CAD build for the part. Positions are in the model's coordinates, mm. A direction names the side the tool comes from. Give positions to 0.01 mm unless a question says otherwise; leave off trailing zeros. Write each loop counter-clockwise with the first axis right and the second up, starting at its lowest first coordinate (ties: lowest second). Pieces come first, ordered by that corner, then holes. Notation, with made-up numbers: (68.25, 27.25) -> (90.25, 27.25) arc R21 ccw to (90.25, 52.25) -> close; hole circle Ø7 at (-23.75, 56.25). An arc over 180 degrees is marked (long way). Answer as a JSON object with one key per item and string values.
```python
from build123d import *

# Parameters (mm, degrees)
BOSS_EXTRUDE1_DEPTH  = 5
EDGE_FLANGE1_START   = -417.4
EDGE_FLANGE1_DEPTH   = 834.8
EDGE_FLANGE1_START_2 = -419.24
EDGE_FLANGE1_2_DEPTH = 838.48
EDGE_FLANGE1_3_DEPTH = 834.8
EDGE_FLANGE1_4_DEPTH = 838.48
BOSS_EXTRUDE2_START  = -20
BOSS_EXTRUDE2_DEPTH  = 20
BOSS_EXTRUDE6_START  = -20
BOSS_EXTRUDE6_DEPTH  = 20
MIRROR2_START        = -20
MIRROR2_COPY_1_DEPTH = 20
MIRROR2_COPY_2_DEPTH = 20
BOSS_EXTRUDE7_DEPTH  = 20
CUT_EXTRUDE1_REACH   = 921.649
SKETCH21_R           = 9.25
BOSS_EXTRUDE8_REACH  = 918.804
SKETCH22_R           = 150
SKETCH23_R           = 145
CUT_EXTRUDE2_DEPTH   = 920.648675088
FILLET1_R            = 10


# Read off the part's stored shape, not the designer's step: Edge-Flange1
with BuildPart() as part:
    # Sketch1 → Boss-Extrude1 (new body)
    with BuildSketch(Plane(origin=(0, 0, 0), x_dir=(1, 0, 0), z_dir=(0, 1, 0))):
        Polygon((-419.24, -417.4), (-419.24, -582.5), (419.24, -582.5), (419.24, -417.4), (482.5, -417.4), (482.5, 417.4), (419.24, 417.4), (419.24, 582.5), (-419.24, 582.5), (-419.24, 417.4), (-482.5, 417.4), (-482.5, -417.4), align=None)
    extrude(amount=BOSS_EXTRUDE1_DEPTH)

    # Edge-Flange1 outline → Edge-Flange1 (add)
    with BuildSketch(Plane.XY.offset(EDGE_FLANGE1_START)):
        with BuildLine():
            Line((-479.84720202, 35.321619656), (-481.510736273, 16.307336141))
            ThreePointArc((-481.510736273, 16.307336141), (-480.800529715, 10.26398325), (-477.748155652, 4.999999958))
            Line((-477.748155652, 4.999999958), (-466.567815802, 5))
            ThreePointArc((-466.567815802, 5), (-473.94058917, 8.244097924), (-476.529762783, 15.871557427))
            Line((-476.529762783, 15.871557427), (-474.86622853, 34.885840943))
            Line((-474.86622853, 34.885840943), (-479.84720202, 35.321619656))
        make_face()
        with BuildLine():
            ThreePointArc((476.529762783, 15.871557427), (473.94058917, 8.244097924), (466.567815802, 5))
            Line((466.567815802, 5), (477.748155652, 4.999999958))
            ThreePointArc((477.748155652, 4.999999958), (480.800529715, 10.26398325), (481.510736273, 16.307336141))
            Line((481.510736273, 16.307336141), (479.84720202, 35.321619656))
            Line((479.84720202, 35.321619656), (474.86622853, 34.885840943))
            Line((474.86622853, 34.885840943), (476.529762783, 15.871557427))
        make_face()
    extrude(amount=EDGE_FLANGE1_DEPTH)

    # Edge-Flange1 2 outline → Edge-Flange1 2 (add)
    with BuildSketch(Plane.YZ.offset(EDGE_FLANGE1_START_2)):
        with BuildLine():
            Line((35.321619656, 579.84720202), (16.307336141, 581.510736273))
            ThreePointArc((16.307336141, 581.510736273), (10.263983245, 580.800529713), (4.99999995, 577.748155645))
            Line((4.99999995, 577.748155645), (5, 566.567815802))
            ThreePointArc((5, 566.567815802), (8.244097924, 573.94058917), (15.871557427, 576.529762783))
            Line((15.871557427, 576.529762783), (34.885840943, 574.86622853))
            Line((34.885840943, 574.86622853), (35.321619656, 579.84720202))
        make_face()
        with BuildLine():
            ThreePointArc((15.871557427, -576.529762783), (8.244097924, -573.94058917), (5, -566.567815802))
            Line((5, -566.567815802), (4.99999995, -577.748155645))
            ThreePointArc((4.99999995, -577.748155645), (10.263983245, -580.800529713), (16.307336141, -581.510736273))
            Line((16.307336141, -581.510736273), (35.321619656, -579.84720202))
            Line((35.321619656, -579.84720202), (34.885840943, -574.86622853))
            Line((34.885840943, -574.86622853), (15.871557427, -576.529762783))
        make_face()
    extrude(amount=EDGE_FLANGE1_2_DEPTH)

    # Edge-Flange1 3 outline → Edge-Flange1 3 (cut)
    with BuildSketch(Plane.XY.offset(EDGE_FLANGE1_START)):
        with BuildLine():
            ThreePointArc((-466.567815802, 0), (-472.691540133, 1.306936051), (-477.748155652, 4.999999958))
            Line((-477.748155652, 4.999999958), (-483, 4.999999958))
            Line((-483, 4.999999958), (-483, -2.2e-08))
            Line((-483, -2.2e-08), (-466.567815802, 0))
        make_face()
        with BuildLine():
            ThreePointArc((477.748155652, 4.999999958), (472.691540133, 1.306936051), (466.567815802, 0))
            Line((466.567815802, 0), (483, -2.2e-08))
            Line((483, -2.2e-08), (483, 4.999999958))
            Line((483, 4.999999958), (477.748155652, 4.999999958))
        make_face()
    extrude(amount=EDGE_FLANGE1_3_DEPTH, mode=Mode.SUBTRACT)

    # Edge-Flange1 4 outline → Edge-Flange1 4 (cut)
    with BuildSketch(Plane.YZ.offset(EDGE_FLANGE1_START_2)):
        with BuildLine():
            ThreePointArc((0, 566.567815802), (1.306936049, 572.691540128), (4.99999995, 577.748155645))
            Line((4.99999995, 577.748155645), (4.99999995, 583))
            Line((4.99999995, 583), (-2.7e-08, 583))
            Line((-2.7e-08, 583), (0, 566.567815802))
        make_face()
        with BuildLine():
            ThreePointArc((4.99999995, -577.748155645), (1.306936049, -572.691540128), (0, -566.567815802))
            Line((0, -566.567815802), (-2.7e-08, -583))
            Line((-2.7e-08, -583), (4.99999995, -583))
            Line((4.99999995, -583), (4.99999995, -577.748155645))
        make_face()
    extrude(amount=EDGE_FLANGE1_4_DEPTH, mode=Mode.SUBTRACT)

    # Sketch18 → Boss-Extrude2 (add)
    with BuildSketch(Plane(origin=(419.24, 0, 0), x_dir=(0, 0, -1), z_dir=(1, 0, 0)).offset(BOSS_EXTRUDE2_START)):
        with BuildLine():
            Line((-417.4, 5), (-566.567815802, 5))
            ThreePointArc((-566.567815802, 5), (-573.94058917, 8.244097924), (-576.529762783, 15.871557427))
            Line((-576.529762783, 15.871557427), (-533.736569049, 505))
            Line((-533.736569049, 505), (-417.4, 505))
            Line((-417.4, 505), (-417.4, 5))
        make_face()
    boss_extrude2 = extrude(amount=BOSS_EXTRUDE2_DEPTH)

    # Sketch19 → Boss-Extrude6 (add)
    with BuildSketch(Plane.XY.offset(417.4).offset(BOSS_EXTRUDE6_START)):
        with BuildLine():
            Line((466.567815802, 5), (419.24, 5))
            Line((419.24, 5), (399.24, 5))
            Line((399.24, 5), (399.24, 505))
            Line((399.24, 505), (419.24, 505))
            Line((419.24, 505), (433.736569049, 505))
            Line((433.736569049, 505), (476.529762783, 15.871557427))
            ThreePointArc((476.529762783, 15.871557427), (473.94058917, 8.244097924), (466.567815802, 5))
        make_face()
    boss_extrude6 = extrude(amount=BOSS_EXTRUDE6_DEPTH)

    # Mirror1: Boss-Extrude2, Boss-Extrude6 across plane
    add(boss_extrude2.mirror(Plane.XY))
    add(boss_extrude6.mirror(Plane.XY))

    # Mirror2: Boss-Extrude2, Boss-Extrude6 across plane
    add(boss_extrude2.mirror(Plane(origin=(0, 0, 0), x_dir=(0, 0, 1), z_dir=(1, 0, 0))))
    add(boss_extrude6.mirror(Plane(origin=(0, 0, 0), x_dir=(0, 0, 1), z_dir=(1, 0, 0))))

    # Mirror2 copy 1 sketch → Mirror2 copy 1 (add)
    with BuildSketch(Plane.ZY.offset(419.24).offset(MIRROR2_START)):
        with BuildLine():
            Line((-417.4, 5), (-566.567815802, 5))
            ThreePointArc((-566.567815802, 5), (-573.94058917, 8.244097924), (-576.529762783, 15.871557427))
            Line((-576.529762783, 15.871557427), (-533.736569049, 505))
            Line((-533.736569049, 505), (-417.4, 505))
            Line((-417.4, 505), (-417.4, 5))
        make_face()
    extrude(amount=MIRROR2_COPY_1_DEPTH)

    # Mirror2 copy 2 sketch → Mirror2 copy 2 (add)
    with BuildSketch(Plane(origin=(0, 0, -417.4), x_dir=(-1, 0, 0), z_dir=(0, 0, -1)).offset(MIRROR2_START)):
        with BuildLine():
            Line((466.567815802, 5), (419.24, 5))
            Line((419.24, 5), (399.24, 5))
            Line((399.24, 5), (399.24, 505))
            Line((399.24, 505), (419.24, 505))
            Line((419.24, 505), (433.736569049, 505))
            Line((433.736569049, 505), (476.529762783, 15.871557427))
            ThreePointArc((476.529762783, 15.871557427), (473.94058917, 8.244097924), (466.567815802, 5))
        make_face()
    extrude(amount=MIRROR2_COPY_2_DEPTH)

    # Sketch20 → Boss-Extrude7 (add)
    with BuildSketch(Plane(origin=(0, 505, 0), x_dir=(1, 0, 0), z_dir=(0, 1, 0))):
        Polygon((-419.24, -417.4), (-419.24, -533.736569049), (419.24, -533.736569049), (419.24, -417.4), (433.736569049, -417.4), (433.736569049, 417.4), (419.24, 417.4), (419.24, 533.736569049), (-419.24, 533.736569049), (-419.24, 417.4), (-433.736569049, 417.4), (-433.736569049, -417.4), align=None)
    extrude(amount=BOSS_EXTRUDE7_DEPTH)

    # Sketch21 → Cut-Extrude1 (cut, up to next)
    with BuildSketch(Plane(origin=(0, 525, 0), x_dir=(1, 0, 0), z_dir=(0, 1, 0)), mode=Mode.PRIVATE) as cut_extrude1_sk1:
        with Locations(Location((0, -249.998440062, 0), (0, 0, 270))):
            Circle(SKETCH21_R)
    cut_extrude1_tool1 = extrude(cut_extrude1_sk1.sketch, amount=-CUT_EXTRUDE1_REACH, mode=Mode.PRIVATE) & part.part
    # Sketch21 → Cut-Extrude1 (cut, up to next)
    with BuildSketch(Plane(origin=(0, 525, 0), x_dir=(1, 0, 0), z_dir=(0, 1, 0)), mode=Mode.PRIVATE) as cut_extrude1_sk2:
        with Locations(Location((-216.505, 124.999220031, 0), (0, 0, 270))):
            Circle(SKETCH21_R)
    cut_extrude1_tool2 = extrude(cut_extrude1_sk2.sketch, amount=-CUT_EXTRUDE1_REACH, mode=Mode.PRIVATE) & part.part
    # Sketch21 → Cut-Extrude1 (cut, up to next)
    with BuildSketch(Plane(origin=(0, 525, 0), x_dir=(1, 0, 0), z_dir=(0, 1, 0)), mode=Mode.PRIVATE) as cut_extrude1_sk3:
        with Locations(Location((216.505, 124.999220031, 0), (0, 0, 270))):
            Circle(SKETCH21_R)
    cut_extrude1_tool3 = extrude(cut_extrude1_sk3.sketch, amount=-CUT_EXTRUDE1_REACH, mode=Mode.PRIVATE) & part.part
    add(cut_extrude1_tool1.solids().sort_by_distance((0, 525, 249.99844))[0], mode=Mode.SUBTRACT)
    add(cut_extrude1_tool2.solids().sort_by_distance((-216.505, 525, -124.99922))[0], mode=Mode.SUBTRACT)
    add(cut_extrude1_tool3.solids().sort_by_distance((216.505, 525, -124.99922))[0], mode=Mode.SUBTRACT)

    # Sketch22 → Boss-Extrude8 (add, up to next)
    with BuildSketch(Plane(origin=(0, 5, 0), x_dir=(1, 0, 0), z_dir=(0, 1, 0)), mode=Mode.PRIVATE) as boss_extrude8_sk1:
        with Locations(Location((0, 0, 0), (0, 0, 270))):
            Circle(SKETCH22_R)
    boss_extrude8_tool1 = extrude(boss_extrude8_sk1.sketch, amount=BOSS_EXTRUDE8_REACH, mode=Mode.PRIVATE) - part.part
    add(boss_extrude8_tool1.solids().sort_by_distance((0, 5, 0))[0])

    # Sketch23 → Cut-Extrude2 (cut, through all)
    with BuildSketch(Plane(origin=(0, 525, 0), x_dir=(1, 0, 0), z_dir=(0, 1, 0))):
        with Locations(Location((0, 0, 0), (0, 0, 270))):
            Circle(SKETCH23_R)
    extrude(amount=-CUT_EXTRUDE2_DEPTH, mode=Mode.SUBTRACT)

    # Fillet1
    fillet1_edges = [part.edges().sort_by_distance(p)[0] for p in [
        (0, 505, -150),
        (0, 5, -150),
    ]]
    fillet(fillet1_edges, radius=FILLET1_R)


solid = part.part
```
1) Slice it at C-C (y = 367.5). List the corners of the cut face in (x, z), then the cut area to 3 significant figures.
Model answer:
{"outline": "(-445.77, -417.4) -> (-419.24, -417.4) -> (-419.24, -545.77) -> (-399.24, -545.77) -> (-399.24, -397.4) -> (-445.77, -397.4) -> close; (-445.77, 397.4) -> (-399.24, 397.4) -> (-399.24, 545.77) -> (-419.24, 545.77) -> (-419.24, 417.4) -> (-445.77, 417.4) -> close; circle Ø300 at (0, 0); (399.24, -545.77) -> (419.24, -545.77) -> (419.24, -417.4) -> (445.77, -417.4) -> (445.77, -397.4) -> (399.24, -397.4) -> close; (399.24, 397.4) -> (445.77, 397.4) -> (445.77, 417.4) -> (419.24, 417.4) -> (419.24, 545.77) -> (399.24, 545.77) -> close; hole circle Ø290 at (0, 0)", "area": "18,600 mm2"}
2) Slice it at A-A (z = -206). List the corners of the cut face in (x, y), then the cut area to 3 significant figures.
Model answer:
{"outline": "(-481.51, 16.31) arc R15 ccw to (-466.57, 0) -> (466.57, 0) arc R15 ccw to (481.51, 16.31) -> (479.85, 35.32) -> (474.87, 34.89) -> (476.53, 15.87) arc R10 cw to (466.57, 5) -> (-466.57, 5) arc R10 cw to (-476.53, 15.87) -> (-474.87, 34.89) -> (-479.85, 35.32) -> close; (-433.74, 505) -> (433.74, 505) -> (433.74, 525) -> (-433.74, 525) -> close", "area": "22,400 mm2"}
3) Mould opens along Z. For faces 3 (the flat face through (419.24, 259, -480)), 4 (the cylindrical face through (43.554, 266.175, 138.304)), 5 (the flat face through (-409.1, 266.65, -554.59)), 6 (the flat face through (-110, 5, -134)) say: released by +Z, released by -Z, zero draft, split by the parting line, or undercut.
Model answer:
{"face 3": "zero draft", "face 4": "undercut", "face 5": "released by -Z", "face 6": "undercut"}
4) Slice it at B-B (x = 270.5). List the corners of the cut face in (y, z).
Model answer:
{"outline": "(0, -566.57) arc R15 ccw to (16.31, -581.51) -> (35.32, -579.85) -> (34.89, -574.87) -> (15.87, -576.53) arc R10 cw to (5, -566.57) -> (5, 566.57) arc R10 cw to (15.87, 576.53) -> (34.89, 574.87) -> (35.32, 579.85) -> (16.31, 581.51) arc R15 ccw to (0, 566.57) -> close; (505, -533.74) -> (525, -533.74) -> (525, 533.74) -> (505, 533.74) -> close"}
5) Slice it at D-D (y = 173). List the corners of the cut face in (x, z).
Model answer:
{"outline": "(-462.78, -417.4) -> (-419.24, -417.4) -> (-419.24, -562.78) -> (-399.24, -562.78) -> (-399.24, -397.4) -> (-462.78, -397.4) -> close; (-462.78, 397.4) -> (-399.24, 397.4) -> (-399.24, 562.78) -> (-419.24, 562.78) -> (-419.24, 417.4) -> (-462.78, 417.4) -> close; circle Ø300 at (0, 0); (399.24, -562.78) -> (419.24, -562.78) -> (419.24, -417.4) -> (462.78, -417.4) -> (462.78, -397.4) -> (399.24, -397.4) -> close; (399.24, 397.4) -> (462.78, 397.4) -> (462.78, 417.4) -> (419.24, 417.4) -> (419.24, 562.78) -> (399.24, 562.78) -> close; hole circle Ø290 at (0, 0)"}
6) 3-axis set-ups, long thin cutter, end or side, ignore diameter. For faces 1 (the flat face through (-419.24, 259, -482)), 2 (the flat face through (-399.24, 252, 486)): which of +Z, -Z, +X, -X, +Y, -Y reach the whole face in a straight line?
Model answer:
{"face 1": "-Z, -X, +Y, -Y", "face 2": "none"}
7) Pin check, flat tips, straight feed: pin 1 (6 mm diameter, centred on x = -127, y = 139, fed in from -Z); pin 2 (1 mm diameter, centred on y = 308.5, z = 14, fed in from +X); pin 3 (16 mm diameter, centred on x = -4.5, y = 513.5, fed in from -Z). Stop position of each tip, or through.
Model answer:
{"pin 1": "stops at z = -84.4", "pin 2": "stops at x = 149.39", "pin 3": "stops at z = -533.74"}
8) Wall check: probe 1 along X at (y, z) = (230.5, 0); probe 2 along Y at (x, z) = (-143, -228.5); probe 3 along X at (y, z) = (465.5, -479). Give the ranges that are in metal, low to high.
Model answer:
{"probe 1": "x = -150 to -145, 145 to 150", "probe 2": "y = 0 to 5, 505 to 525", "probe 3": "x = -419.24 to -399.24, 399.24 to 419.24"}
